Can you work these out from the model? Positions are in its coordinate system, mm. Face numbers are marked on the shaded views. A direction names the side the tool comes from. Round coordinates to 2 decimals unless told otherwise and drop trailing zeros. Write each loop counter-clockwise with the first axis right and the second up, starting at its lowest first coordinate (ties: lowest second). Pieces come first, ordered by that corner, then holes. Notation, with made-up numbers: (70, 37.25) -> (116, 37.25) arc R32 ccw to (116, 66.25) -> close; hole circle Ø10 at (-23, 79). An arc over 180 degrees is marked (long way). Use CSV: the item, a comma, the result in double quotes.
```python
from build123d import *

# Parameters (mm, degrees)
CYLINDER017_R               = 2.8
CYLINDER017_DEPTH           = 60
CYLINDER016_R               = 2.8
CYLINDER016_DEPTH           = 60
CYLINDER022_R               = 2.8
CYLINDER022_DEPTH           = 60
CYLINDER021_R               = 2.8
CYLINDER021_DEPTH           = 60
CYLINDER026_R               = 4.75
CYLINDER026_DEPTH           = 16
CYLINDER026_ROLL_ANGLE      = -89.999776
CYLINDER026_PITCH_ANGLE     = 1.4e-05
CYLINDER026_PLACEMENT_ANGLE = -9.999925
PAD006_DEPTH                = 47


with BuildPart() as u006:
    # Cylinder017 → Cylinder017 (new body)
    with BuildSketch(Plane(origin=(41, -20, -3), x_dir=(0, 0, 1), z_dir=(-1, 0, 0))):
        Circle(CYLINDER017_R)
    extrude(amount=CYLINDER017_DEPTH)


with BuildPart() as u005:
    # Cylinder016 → Cylinder016 (new body)
    with BuildSketch(Plane(origin=(41, -4, -3), x_dir=(0, 0, 1), z_dir=(-1, 0, 0))):
        Circle(CYLINDER016_R)
    extrude(amount=CYLINDER016_DEPTH)


with BuildPart() as o006:
    # Cylinder022 → Cylinder022 (new body)
    with BuildSketch(Plane(origin=(41, -4, 36), x_dir=(0, 0, 1), z_dir=(-1, 0, 0))):
        Circle(CYLINDER022_R)
    extrude(amount=CYLINDER022_DEPTH)


with BuildPart() as o005:
    # Cylinder021 → Cylinder021 (new body)
    with BuildSketch(Plane(origin=(41, -20, 36), x_dir=(0, 0, 1), z_dir=(-1, 0, 0))):
        Circle(CYLINDER021_R)
    extrude(amount=CYLINDER021_DEPTH)


with BuildPart() as cylinder026:
    # Cylinder026 → Cylinder026 (new body)
    with BuildSketch(Plane.XY):
        Circle(CYLINDER026_R)
    extrude(amount=CYLINDER026_DEPTH)


with BuildPart() as cylinder026_1:
    # Cylinder026 roll: moved
    add(cylinder026.part.rotate(Axis((0, 0, 0), (1, 0, 0)), CYLINDER026_ROLL_ANGLE))


with BuildPart() as cylinder026_2:
    # Cylinder026 pitch: moved
    add(cylinder026_1.part.rotate(Axis((0, 0, 0), (0, 1, 0)), CYLINDER026_PITCH_ANGLE))


with BuildPart() as cylinder026_3:
    # Cylinder026 placement: moved
    add(cylinder026_2.part.moved(Location((33.913531, -36.278084, 16.499961))).rotate(Axis((33.913531, -36.278084, 16.499961), (0, 0, 1)), CYLINDER026_PLACEMENT_ANGLE))


with BuildPart() as cut027:
    # Sketch006 → Pad006 (new body)
    with BuildSketch(Plane.XY):
        Polygon((29.25, 0), (25.25, 0), (25.25, -28), (44.946155, -31.472964), (45.640748, -27.533733), (29.25, -24.643601), align=None)
    extrude(amount=PAD006_DEPTH)


with BuildPart() as cut027_1:
    # Body006 placement: moved
    add(cut027.part.moved(Location((0, 0, -7))))

    # Cut021: cut Cylinder026
    add(cylinder026_3.part, mode=Mode.SUBTRACT)

    # Cut024: cut O005
    add(o005.part, mode=Mode.SUBTRACT)

    # Cut025: cut O006
    add(o006.part, mode=Mode.SUBTRACT)

    # Cut026: cut U005
    add(u005.part, mode=Mode.SUBTRACT)

    # Cut027: cut U006
    add(u006.part, mode=Mode.SUBTRACT)


solid = cut027_1.part
```
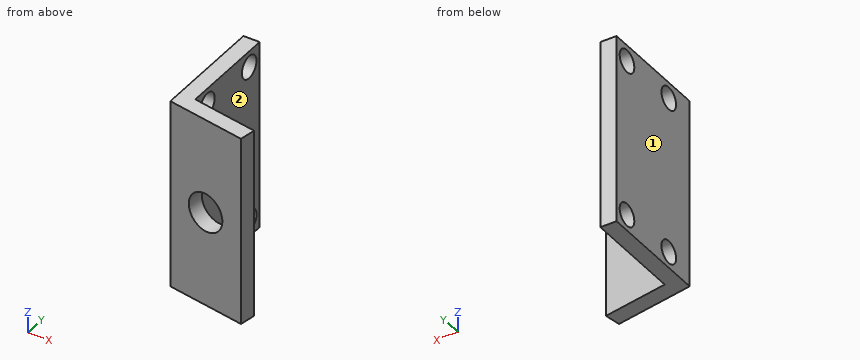
Q1. Suppose I cut it at B-B (z = -3). Write out the boundary of the cut face in (x, y), and give its area (3 significant figures).
Resolved:
outline,"(25.25, -28) -> (44.95, -31.47) -> (45.64, -27.53) -> (29.25, -24.64) -> (29.25, -22.8) -> (25.25, -22.8) -> close; (25.25, -17.2) -> (29.25, -17.2) -> (29.25, -6.8) -> (25.25, -6.8) -> close; (25.25, -1.2) -> (29.25, -1.2) -> (29.25, 0) -> (25.25, 0) -> close"
area,"134 mm^2"
Q2. Suppose I cut it at C-C (z = 25). Write out the boundary of the cut face in (x, y), and give its area (3 significant figures).
Resolved:
outline,"(25.25, -28) -> (44.95, -31.47) -> (45.64, -27.53) -> (29.25, -24.64) -> (29.25, 0) -> (25.25, 0) -> close"
area,"179 mm^2"
Q3. Suppose I cut it at D-D (y = -10.5). Write out the boundary of the cut face in (x, z), and give its area (3 significant figures).
Resolved:
outline,"(25.25, -7) -> (29.25, -7) -> (29.25, 40) -> (25.25, 40) -> close"
area,"188 mm^2"
Q4. Please list where these lines run through material, in increasing order: probe 1 along Z at (x, y) = (27.15, -4); probe 2 along Y at (x, z) = (26.6, -3); probe 3 along Y at (x, z) = (27.85, -3).
Resolved:
probe 1,"z = -7 to -5.8, -0.2 to 33.2, 38.8 to 40"
probe 2,"y = -28.24 to -22.8, -17.2 to -6.8, -1.2 to 0"
probe 3,"y = -28.46 to -22.8, -17.2 to -6.8, -1.2 to 0"
Q5. Suppose I cut it at A-A (y = -4). Write out the boundary of the cut face in (x, z).
Resolved:
outline,"(25.25, -7) -> (29.25, -7) -> (29.25, -5.8) -> (25.25, -5.8) -> close; (25.25, -0.2) -> (29.25, -0.2) -> (29.25, 33.2) -> (25.25, 33.2) -> close; (25.25, 38.8) -> (29.25, 38.8) -> (29.25, 40) -> (25.25, 40) -> close"
Q6. On a 3-axis mill with a long thin cutter (end or side, diameter ignored), from which of +Z, -Z, +X, -X, +Y, -Y can I reach the whole of each face in a straight line? I mean the marked faces 1 and 2. Say none if no direction works.
Resolved:
face 1,"+Z, -Z, -X, +Y, -Y"
face 2,"+Z, -Z, +X, +Y"
Q7. Will these pins go through, and if not, where does the flat tip stop? P1, Ø9, axis at y = -4, z = 36, coming from the +X side; P2, Ø2, axis at x = 42, z = 17.5, coming from the +Y side; P3, Ø6, axis at x = 28, z = -1.5, coming from the +Y side; P4, Ø6, axis at x = 28.5, z = 26, coming from the -Y side.
Resolved:
P1,"stops at x = 29.25"
P2,"stops at y = -26.72"
P3,"stops at y = 0"
P4,"stops at y = -29.1"
